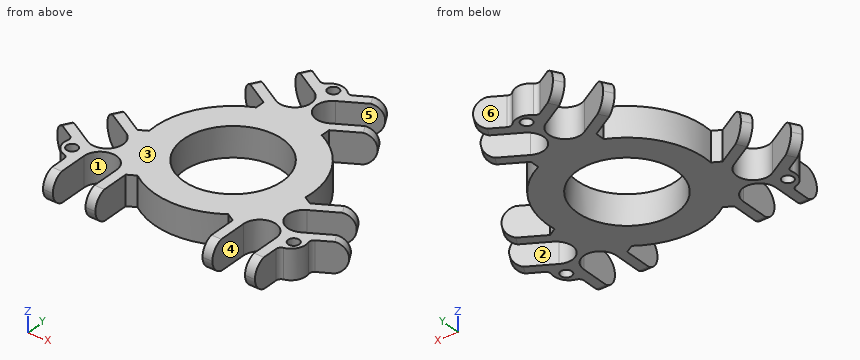
```python
from build123d import *

# Parameters (mm, degrees)
F0_R          = 2.25
F0_R_2        = 20
F1_DEPTH      = 12
F5_DEPTH      = 25
F5_DEPTH_BACK = 68
F6_DEPTH      = 25
F6_DEPTH_BACK = 68
F7_DEPTH      = 25
F7_DEPTH_BACK = 68


with BuildPart() as f1:
    # F0 (on Top) → F1 (new body)
    with BuildSketch(Plane.XY):
        with BuildLine():
            Line((-13.2341793977, 32.6400236937), (-13.2341793977, 28.8603360284))
            ThreePointArc((-13.2341793977, 28.8603360284), (-27.4963065702, 15.875), (-31.6108738612, -2.9690324575))
            Line((-31.6108738612, -2.9690324575), (-34.8841793977, -4.8588762902))
            Line((-34.8841793977, -4.8588762902), (-48.4064064606, 2.9481851446))
            Line((-48.4064064606, 2.9481851446), (-50.4064064606, -0.5159164705))
            Line((-50.4064064606, -0.5159164705), (-36.55, -8.5159164705))
            ThreePointArc((-36.55, -8.5159164705), (-34.134232335, -17.5316841355), (-43.15, -19.9474518005))
            Line((-43.15, -19.9474518005), (-57.0064064606, -11.9474518005))
            Line((-57.0064064606, -11.9474518005), (-59.0064064606, -15.4115534156))
            Line((-59.0064064606, -15.4115534156), (-49.5582039325, -20.8664756886))
            ThreePointArc((-49.5582039325, -20.8664756886), (-48.7069743457, -21.8415925381), (-48.6311529494, -23.1337596308))
            ThreePointArc((-48.6311529494, -23.1337596308), (-48.0461524227, -27.7394590348), (-44.35, -30.5489340541))
            ThreePointArc((-44.35, -30.5489340541), (-43.2688611699, -31.2606808558), (-42.85, -32.4854257272))
            Line((-42.85, -32.4854257272), (-42.85, -43.395270273))
            Line((-42.85, -43.395270273), (-38.85, -43.395270273))
            Line((-38.85, -43.395270273), (-38.85, -27.395270273))
            ThreePointArc((-38.85, -27.395270273), (-32.25, -20.795270273), (-25.65, -27.395270273))
            Line((-25.65, -27.395270273), (-25.65, -43.395270273))
            Line((-25.65, -43.395270273), (-21.65, -43.395270273))
            Line((-21.65, -43.395270273), (-21.65, -27.7811474035))
            Line((-21.65, -27.7811474035), (-18.3766944635, -25.8913035708))
            ThreePointArc((-18.3766944635, -25.8913035708), (0, -31.75), (18.3766944635, -25.8913035708))
            Line((18.3766944635, -25.8913035708), (21.65, -27.7811474035))
            Line((21.65, -27.7811474035), (21.65, -43.395270273))
            Line((21.65, -43.395270273), (25.65, -43.395270273))
            Line((25.65, -43.395270273), (25.65, -27.395270273))
            ThreePointArc((25.65, -27.395270273), (32.25, -20.795270273), (38.85, -27.395270273))
            Line((38.85, -27.395270273), (38.85, -43.395270273))
            Line((38.85, -43.395270273), (42.85, -43.395270273))
            Line((42.85, -43.395270273), (42.85, -32.4854257272))
            ThreePointArc((42.85, -32.4854257272), (43.2688611699, -31.2606808558), (44.35, -30.5489340541))
            ThreePointArc((44.35, -30.5489340541), (48.0461524227, -27.7394590348), (48.6311529494, -23.1337596308))
            ThreePointArc((48.6311529494, -23.1337596308), (48.7069743457, -21.8415925381), (49.5582039325, -20.8664756886))
            Line((49.5582039325, -20.8664756886), (59.0064064606, -15.4115534156))
            Line((59.0064064606, -15.4115534156), (57.0064064606, -11.9474518005))
            Line((57.0064064606, -11.9474518005), (43.15, -19.9474518005))
            ThreePointArc((43.15, -19.9474518005), (34.134232335, -17.5316841355), (36.55, -8.5159164705))
            Line((36.55, -8.5159164705), (50.4064064606, -0.5159164705))
            Line((50.4064064606, -0.5159164705), (48.4064064606, 2.9481851446))
            Line((48.4064064606, 2.9481851446), (34.8841793977, -4.8588762902))
            Line((34.8841793977, -4.8588762902), (31.6108738612, -2.9690324575))
            ThreePointArc((31.6108738612, -2.9690324575), (27.4963065702, 15.875), (13.2341793977, 28.8603360284))
            Line((13.2341793977, 28.8603360284), (13.2341793977, 32.6400236937))
            Line((13.2341793977, 32.6400236937), (26.7564064606, 40.4470851285))
            Line((26.7564064606, 40.4470851285), (24.7564064606, 43.9111867436))
            Line((24.7564064606, 43.9111867436), (10.9, 35.9111867436))
            ThreePointArc((10.9, 35.9111867436), (1.884232335, 38.3269544086), (4.3, 47.3427220735))
            Line((4.3, 47.3427220735), (18.1564064606, 55.3427220735))
            Line((18.1564064606, 55.3427220735), (16.1564064606, 58.8068236887))
            Line((16.1564064606, 58.8068236887), (6.7082039325, 53.3519014158))
            ThreePointArc((6.7082039325, 53.3519014158), (5.4381131758, 53.1022733939), (4.2811529494, 53.6826936849))
            ThreePointArc((4.2811529494, 53.6826936849), (0, 55.4789180696), (-4.2811529494, 53.6826936849))
            ThreePointArc((-4.2811529494, 53.6826936849), (-5.4381131758, 53.1022733939), (-6.7082039325, 53.3519014158))
            Line((-6.7082039325, 53.3519014158), (-16.1564064606, 58.8068236887))
            Line((-16.1564064606, 58.8068236887), (-18.1564064606, 55.3427220735))
            Line((-18.1564064606, 55.3427220735), (-4.3, 47.3427220735))
            ThreePointArc((-4.3, 47.3427220735), (-1.884232335, 38.3269544086), (-10.9, 35.9111867436))
            Line((-10.9, 35.9111867436), (-24.7564064606, 43.9111867436))
            Line((-24.7564064606, 43.9111867436), (-26.7564064606, 40.4470851285))
            Line((-26.7564064606, 40.4470851285), (-13.2341793977, 32.6400236937))
        make_face()
        with Locations((-44.8037193958, -25.8674394539)):
            Circle(F0_R, mode=Mode.SUBTRACT)
        with Locations((44.8037193958, -25.8674394539)):
            Circle(F0_R, mode=Mode.SUBTRACT)
        Circle(F0_R_2, mode=Mode.SUBTRACT)
        with Locations((0, 51.7348789078)):
            Circle(F0_R, mode=Mode.SUBTRACT)
    extrude(amount=F1_DEPTH)

    # F2 (on face) → F5 (cut, two sides)
    with BuildSketch(Plane(origin=(21.65, 0, 0), x_dir=(0, -1, 0), z_dir=(-1, 0, 0))) as f5_sk:
        with BuildLine():
            ThreePointArc((38.7840602421, 12), (42.1092993822, 9.7836245172), (43.395270273, 6))
            Line((43.395270273, 6), (43.395270273, 12))
            Line((43.395270273, 12), (38.7840602421, 12))
        make_face()
        with BuildLine():
            ThreePointArc((38.7840602421, 0), (38.0044089294, -0.1549812), (37.2113464037, -0.2090845469))
            Line((37.2113464037, -0.2090845469), (37.2113464037, -2.7538968716))
            Line((37.2113464037, -2.7538968716), (50.0447638333, -2.7538968716))
            Line((50.0447638333, -2.7538968716), (50.0447638333, 14.7538968716))
            Line((50.0447638333, 14.7538968716), (37.2113464037, 14.7538968716))
            Line((37.2113464037, 14.7538968716), (37.2113464037, 12.2090845469))
            ThreePointArc((37.2113464037, 12.2090845469), (38.0044089294, 12.1549812), (38.7840602421, 12))
            Line((38.7840602421, 12), (43.395270273, 12))
            Line((43.395270273, 12), (43.395270273, 6))
            Line((43.395270273, 6), (43.395270273, 0))
            Line((43.395270273, 0), (38.7840602421, 0))
        make_face()
        with BuildLine():
            ThreePointArc((43.395270273, 6), (42.1092993822, 2.2163754828), (38.7840602421, 0))
            Line((38.7840602421, 0), (43.395270273, 0))
            Line((43.395270273, 0), (43.395270273, 6))
        make_face()
    extrude(amount=-F5_DEPTH, mode=Mode.SUBTRACT)
    extrude(f5_sk.sketch, amount=F5_DEPTH_BACK, mode=Mode.SUBTRACT)

    # F3 (on face) → F6 (cut, two sides)
    with BuildSketch(Plane(origin=(-10.825, 18.7494499919, 0), x_dir=(0.8660254038, 0.5, 0), z_dir=(0.5, -0.8660254038, 0))) as f6_sk:
        with BuildLine():
            ThreePointArc((38.7840602421, 0), (38.0044089294, -0.1549812), (37.2113464037, -0.2090845469))
            Line((37.2113464037, -0.2090845469), (37.2113464037, -2.7538968716))
            Line((37.2113464037, -2.7538968716), (50.0447638333, -2.7538968716))
            Line((50.0447638333, -2.7538968716), (50.0447638333, 14.7538968716))
            Line((50.0447638333, 14.7538968716), (37.2113464037, 14.7538968716))
            Line((37.2113464037, 14.7538968716), (37.2113464037, 12.2090845469))
            ThreePointArc((37.2113464037, 12.2090845469), (38.0044089294, 12.1549812), (38.7840602421, 12))
            Line((38.7840602421, 12), (43.395270273, 12))
            Line((43.395270273, 12), (43.395270273, 6))
            Line((43.395270273, 6), (43.395270273, 0))
            Line((43.395270273, 0), (38.7840602421, 0))
        make_face()
        with BuildLine():
            ThreePointArc((38.7840602421, 12), (42.1092993822, 9.7836245172), (43.395270273, 6))
            Line((43.395270273, 6), (43.395270273, 12))
            Line((43.395270273, 12), (38.7840602421, 12))
        make_face()
        with BuildLine():
            ThreePointArc((43.395270273, 6), (42.1092993822, 2.2163754828), (38.7840602421, 0))
            Line((38.7840602421, 0), (43.395270273, 0))
            Line((43.395270273, 0), (43.395270273, 6))
        make_face()
    extrude(amount=-F6_DEPTH, mode=Mode.SUBTRACT)
    extrude(f6_sk.sketch, amount=F6_DEPTH_BACK, mode=Mode.SUBTRACT)

    # F4 (on face) → F7 (cut, two sides)
    with BuildSketch(Plane(origin=(-10.825, -18.7494499919, 0), x_dir=(-0.8660254038, 0.5, 0), z_dir=(0.5, 0.8660254038, 0))) as f7_sk:
        with BuildLine():
            ThreePointArc((38.7840602421, 0), (38.0044089294, -0.1549812), (37.2113464037, -0.2090845469))
            Line((37.2113464037, -0.2090845469), (37.2113464037, -2.7538968716))
            Line((37.2113464037, -2.7538968716), (50.0447638333, -2.7538968716))
            Line((50.0447638333, -2.7538968716), (50.0447638333, 14.7538968716))
            Line((50.0447638333, 14.7538968716), (37.2113464037, 14.7538968716))
            Line((37.2113464037, 14.7538968716), (37.2113464037, 12.2090845469))
            ThreePointArc((37.2113464037, 12.2090845469), (38.0044089294, 12.1549812), (38.7840602421, 12))
            Line((38.7840602421, 12), (43.395270273, 12))
            Line((43.395270273, 12), (43.395270273, 6))
            Line((43.395270273, 6), (43.395270273, 0))
            Line((43.395270273, 0), (38.7840602421, 0))
        make_face()
        with BuildLine():
            ThreePointArc((43.395270273, 6), (42.1092993822, 2.2163754828), (38.7840602421, 0))
            Line((38.7840602421, 0), (43.395270273, 0))
            Line((43.395270273, 0), (43.395270273, 6))
        make_face()
        with BuildLine():
            ThreePointArc((38.7840602421, 12), (42.1092993822, 9.7836245172), (43.395270273, 6))
            Line((43.395270273, 6), (43.395270273, 12))
            Line((43.395270273, 12), (38.7840602421, 12))
        make_face()
    extrude(amount=-F7_DEPTH, mode=Mode.SUBTRACT)
    extrude(f7_sk.sketch, amount=F7_DEPTH_BACK, mode=Mode.SUBTRACT)


solid = f1.part
```
The model under review builds one solid part; all positions refer to its coordinate system, in mm. Face numbers are marked on the shaded views. A direction names the side the tool comes from. Round coordinates to 2 decimals unless told otherwise and drop trailing zeros. Write each loop counter-clockwise with the first axis right and the second up, starting at its lowest first coordinate (ties: lowest second). Pieces come first, ordered by that corner, then holes. Notation, with made-up numbers: (2, 15.25) - (43, 15.25) arc R20 cw to (43, 47.25) - close; hole circle Ø7 at (-30, 7.5). An arc over 180 degrees is marked (long way). Use one line per item in the form item = value.
Q1. Consider section B-B (z = 2). State how many separate pieces and enclosed holes the cut face has, and give its area (3 significant figures).
Answer key:
separate_pieces = 1
enclosed_holes = 4
area = 3,230 mm2
Q2. Insertion check: pin 1 Ø6 at (y, z) = (-36.5, 6) entering from +X; pin 2 Ø6 at (y, z) = (-33, 8.5) entering from +X; pin 3 Ø3 at (y, z) = (-29, 1.5) entering from +X. Each pin has a flat end and moves straight along its axis. Give the tip position at first contact, or say it passes through.
Answer key:
pin_1 = 42.85
pin_2 = 45.74
pin_3 = 48.18
Q3. Consider section A-A (y = 17). State the section outline as (x, z) points.
Answer key:
outline = (-26.82, 0) - (-10.54, 0) - (-10.54, 12) - (-26.82, 12) - close; (10.54, 0) - (26.82, 0) - (26.82, 12) - (10.54, 12) - close
Q4. Tool access review of the marked faces 4, 5 and 6: name each direction out of +Z, -Z, +X, -X, +Y, -Y from which nothing blocks a thin tool from reaching the whole face with its end or side.
Answer key:
face_4 = +Z, -Z, -Y
face_5 = +Z, -Z, +X
face_6 = +Z, -Z, +Y
Q5. For line 1 (X direction, y = -33.5, z = 5); line 2 (X direction, y = -25, z = 3); line 3 (Y direction, x = -14.5, z = 2.5), list the stretches that pass through material, from the lowest coordinate up. Write a range as [from, to].
Answer key:
line_1 = [-42.85, -38.85], [-25.65, -21.65], [21.65, 25.65], [38.85, 42.85]
line_2 = [-48.84, -46.88], [-42.73, -38.4], [-26.1, 26.1], [38.4, 42.73], [46.88, 48.84]
line_3 = [-28.25, -13.77], [13.77, 28.25], [33.37, 37.99], [53.23, 57.85]
Q6. Draft analysis for pull direction Y (two halves, no side actions). For the marked faces 1, 2 and 3, state which applies: +Y half, -Y half, draft (parallel to the pull), parting line (faces both ways), or undercut.
Answer key:
face_1 = -Y half
face_2 = undercut
face_3 = draft
